Build history of the part. All positions in model axes, mm. Give positions to 0.01 mm unless a question says otherwise; leave off trailing zeros. Order: outer loops, then holes, each group sorted by start corner. A loop starts at its lowest first (then second) coordinate and runs counter-clockwise, first axis right, second up. Notation, with made-up numbers: (-31.75, 55) -> (14.25, 55) arc R8 cw to (14.25, 62) -> close; hole circle Ø10 at (-11.75, 75). An arc over 180 degrees is marked (long way). Use a Markdown table: item, result. Add a question column.
```python
from build123d import *

# Parameters (mm, degrees)
SKETCH1_R           = 17.5
SKETCH1_R_2         = 3.875
SKETCH1_R_3         = 0.8
BOSS_EXTRUDE1_DEPTH = 1.825


with BuildPart() as part:
    # Sketch1 → Boss-Extrude1 (new, symmetric)
    with BuildSketch(Plane.XY):
        Circle(SKETCH1_R)
        Circle(SKETCH1_R_2, mode=Mode.SUBTRACT)
        with Locations((7.75, 0)):
            Circle(SKETCH1_R_3, mode=Mode.SUBTRACT)
        with Locations((0, 7.75)):
            Circle(SKETCH1_R_3, mode=Mode.SUBTRACT)
        with Locations(Location((-7.75, 0, 0), (0, 0, 180))):
            Circle(SKETCH1_R_3, mode=Mode.SUBTRACT)
        with Locations(Location((0, -7.75, 0), (0, 0, 180))):
            Circle(SKETCH1_R_3, mode=Mode.SUBTRACT)
    extrude(amount=BOSS_EXTRUDE1_DEPTH, both=True)


solid = part.part
```
(1) Mould opens along Y. For faces 1 (the face through (-13.887, -10.648, 0.026)), 2 (the face through (-0.2, 4.1, 1.825)), 3 (the face through (-0.104, 8.543, -0.026)) say: released by +Y, released by -Y, zero draft, split by the parting line, or undercut.
(2) Pin check, flat tips, straight feed: pin 1 Ø1.3 at (x, y) = (-7.75, 0) entering from +Z; pin 2 Ø12.5 at (x, y) = (0, 0) entering from -Z (3 decimals); pin 3 Ø2 at (x, z) = (-3, 0) entering from +Y; pin 4 Ø1 at (y, z) = (-13.5, 0) entering from -X. Stop position of each tip, or through.
(3) Band-saw the part on A-A on x = 0. Give the cut face in (y, z) (3 decimals).
(4) Band-saw the part on C-C on z = 0.9. Give the cut face in (x, y) (3 decimals), plus the area to 3 significant figures.
(5) Wall check: probe 1 along Y at (x, z) = (0, -1.65) (3 decimals); probe 2 along X at (y, z) = (-0.5, -0.65); probe 3 along X at (y, z) = (-1.5, 0.9). Give the ranges that are in metal, low to high.
(6) Band-saw the part on D-D on y = -7.75. Give the cut face in (x, z) (3 decimals).
Response:
| question | item | result |
|---|---|---|
| 1 | face 1 | split by the parting line |
| 1 | face 2 | zero draft |
| 1 | face 3 | undercut |
| 2 | pin 1 | passes through |
| 2 | pin 2 | stops at z = -1.825 |
| 2 | pin 3 | stops at y = 17.39 |
| 2 | pin 4 | stops at x = -11.72 |
| 3 | outline | (-17.5, -1.825) -> (-8.55, -1.825) -> (-8.55, 1.825) -> (-17.5, 1.825) -> close; (-6.95, -1.825) -> (-3.875, -1.825) -> (-3.875, 1.825) -> (-6.95, 1.825) -> close; (3.875, -1.825) -> (6.95, -1.825) -> (6.95, 1.825) -> (3.875, 1.825) -> close; (8.55, -1.825) -> (17.5, -1.825) -> (17.5, 1.825) -> (8.55, 1.825) -> close |
| 4 | outline | circle Ø35 at (0, 0); hole circle Ø1.6 at (-7.75, 0); hole circle Ø7.75 at (0, 0); hole circle Ø1.6 at (0, -7.75); hole circle Ø1.6 at (0, 7.75); hole circle Ø1.6 at (7.75, 0) |
| 4 | area | 907 mm² |
| 5 | probe 1 | y = -17.5 to -8.55, -6.95 to -3.875, 3.875 to 6.95, 8.55 to 17.5 |
| 5 | probe 2 | x = -17.49 to -8.37, -7.13 to -3.84, 3.84 to 7.13, 8.37 to 17.49 |
| 5 | probe 3 | x = -17.44 to -3.57, 3.57 to 17.44 |
| 6 | outline | (-15.69, -1.825) -> (-0.8, -1.825) -> (-0.8, 1.825) -> (-15.69, 1.825) -> close; (0.8, -1.825) -> (15.69, -1.825) -> (15.69, 1.825) -> (0.8, 1.825) -> close |
